For this review, take the finished solid that the model builds, in its own axes (mm). Round coordinates to 2 decimals unless told otherwise and drop trailing zeros. Order: outer loops, then holes, each group sorted by start corner. A loop starts at its lowest first (then second) coordinate and runs counter-clockwise, first axis right, second up. Notation, with made-up numbers: M 8.25,86.5 L 31.25,86.5 A31 ccw 31.25,125.5 Z; hole C -13.5,-35 d3. An arc over 180 degrees is marked long. Answer as a JSON object with one key per item and string values.
from build123d import *

# Parameters (mm, degrees)
SZKIC1_R                    = 10
DODANIE_WYCI_GNI_CIE1_DEPTH = 2


with BuildPart() as part:
    # Szkic1 → Dodanie-wyciągnięcie1 (new body)
    with BuildSketch(Plane(origin=(0, 0, 0), x_dir=(1, 0, 0), z_dir=(0, 1, 0))):
        with BuildLine():
            Line((25.724787771, -25.724787771), (23.475270357, -18.679177757))
            ThreePointArc((23.475270357, -18.679177757), (30, 0), (23.475270357, 18.679177757))
            Line((23.475270357, 18.679177757), (25.724787771, 25.724787771))
            Line((25.724787771, 25.724787771), (8.05822964, 29.607826273))
            add(Edge.make_bspline(
                [(8.05822964, 29.607826273), (7.79792239, 31.378992774), (7.507535684, 33.029118956)],
                knots=[5.346121376, 5.346121376, 5.346121376, 5.433983203, 5.433983203, 5.433983203], degree=2, weights=[1, 0.999035193, 1]))
            add(Edge.make_bspline(
                [(7.507535684, 33.029118956), (5.218865934, 46.034514162), (1.811566447, 49.17271271)],
                knots=[5.433983203, 5.433983203, 5.433983203, 6.101022879, 6.101022879, 6.101022879], degree=2, weights=[1, 0.944895907, 1]))
            add(Edge.make_bspline(
                [(1.811566447, 49.17271271), (0.913339162, 50), (0, 50)],
                knots=[6.101022879, 6.101022879, 6.101022879, 6.283185307, 6.283185307, 6.283185307], degree=2, weights=[1, 0.995854973, 1]))
            add(Edge.make_bspline(
                [(0, 50), (-0.913339162, 50), (-1.811566447, 49.17271271)],
                knots=[0, 0, 0, 0.182162428, 0.182162428, 0.182162428], degree=2, weights=[1, 0.995854973, 1]))
            add(Edge.make_bspline(
                [(-1.811566447, 49.17271271), (-5.218865934, 46.034514162), (-7.507535684, 33.029118956)],
                knots=[0.182162428, 0.182162428, 0.182162428, 0.849202104, 0.849202104, 0.849202104], degree=2, weights=[1, 0.944895907, 1]))
            add(Edge.make_bspline(
                [(-7.507535684, 33.029118956), (-7.79792239, 31.378992774), (-8.05822964, 29.607826273)],
                knots=[0.849202104, 0.849202104, 0.849202104, 0.937063931, 0.937063931, 0.937063931], degree=2, weights=[1, 0.999035193, 1]))
            Line((-8.05822964, 29.607826273), (-25.724787771, 25.724787771))
            Line((-25.724787771, 25.724787771), (-23.475270357, 18.679177757))
            ThreePointArc((-23.475270357, 18.679177757), (-30, 0), (-23.475270357, -18.679177757))
            Line((-23.475270357, -18.679177757), (-25.724787771, -25.724787771))
            Line((-25.724787771, -25.724787771), (-8.05822964, -29.607826273))
            add(Edge.make_bspline(
                [(-8.05822964, -29.607826273), (-7.79792239, -31.378992774), (-7.507535684, -33.029118956)],
                knots=[2.204528722, 2.204528722, 2.204528722, 2.292390549, 2.292390549, 2.292390549], degree=2, weights=[1, 0.999035193, 1]))
            add(Edge.make_bspline(
                [(-7.507535684, -33.029118956), (-5.218865934, -46.034514162), (-1.811566447, -49.17271271)],
                knots=[2.292390549, 2.292390549, 2.292390549, 2.959430225, 2.959430225, 2.959430225], degree=2, weights=[1, 0.944895907, 1]))
            add(Edge.make_bspline(
                [(-1.811566447, -49.17271271), (-0.913339162, -50), (0, -50)],
                knots=[2.959430225, 2.959430225, 2.959430225, 3.141592654, 3.141592654, 3.141592654], degree=2, weights=[1, 0.995854973, 1]))
            add(Edge.make_bspline(
                [(0, -50), (0.913339162, -50), (1.811566447, -49.17271271)],
                knots=[3.141592654, 3.141592654, 3.141592654, 3.323755082, 3.323755082, 3.323755082], degree=2, weights=[1, 0.995854973, 1]))
            add(Edge.make_bspline(
                [(1.811566447, -49.17271271), (5.218865934, -46.034514162), (7.507535684, -33.029118956)],
                knots=[3.323755082, 3.323755082, 3.323755082, 3.990794758, 3.990794758, 3.990794758], degree=2, weights=[1, 0.944895907, 1]))
            add(Edge.make_bspline(
                [(7.507535684, -33.029118956), (7.79792239, -31.378992774), (8.05822964, -29.607826273)],
                knots=[3.990794758, 3.990794758, 3.990794758, 4.078656585, 4.078656585, 4.078656585], degree=2, weights=[1, 0.999035193, 1]))
            Line((8.05822964, -29.607826273), (25.724787771, -25.724787771))
        make_face()
        with Locations(Location((0, 0, 0), (0, 0, 270))):
            Circle(SZKIC1_R, mode=Mode.SUBTRACT)
    extrude(amount=DODANIE_WYCI_GNI_CIE1_DEPTH)


solid = part.part
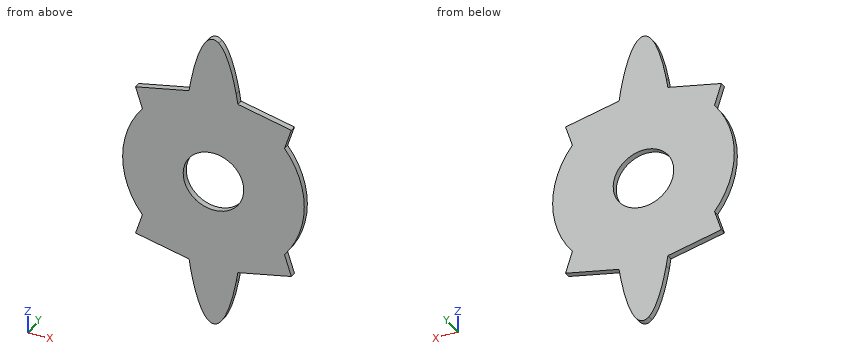
1) Add section C-C on x = 21.5. State the section outline as (y, z) points, and give its area (3 significant figures).
Geometry check:
{"outline": "M 0,-26.65 L 2,-26.65 L 2,26.65 L 0,26.65 Z", "area": "107 mm²"}
2) For L1, parallel to X at y = 1.3, z = 0; L2, parallel to X at y = 1.15, z = 6.5; L3, parallel to Z at x = -3.5, y = 1.6, list the stretches that pass through material, from the lowest coordinate up.
Geometry check:
{"L1": "x = -30 to -10, 10 to 30", "L2": "x = -29.29 to -7.6, 7.6 to 29.29", "L3": "z = -46.84 to -9.37, 9.37 to 46.84"}
3) Add section A-A on z = 0. State the section outline as (x, y) points.
Geometry check:
{"outline": "M -30,0 L -10,0 L -10,2 L -30,2 Z; M 10,0 L 30,0 L 30,2 L 10,2 Z"}
4) Add section B-B on z = -20.5. State the section outline as (x, y) points, and give its area (3 significant figures).
Geometry check:
{"outline": "M -24.06,0 L 24.06,0 L 24.06,2 L -24.06,2 Z", "area": "96.2 mm²"}
